Read the model definition and answer for the solid it produces. Units are mm, in the model's axes. Face numbers are marked on the shaded views. A direction names the side the tool comes from. Coordinates: 2 decimals unless noted, no trailing zeros. Order: outer loops, then holes, each group sorted by start corner. A loop starts at its lowest first (then second) coordinate and runs counter-clockwise, first axis right, second up. Notation, with made-up numbers: (73.25, -14) - (129.25, -14) arc R12 ccw to (129.25, -5) - close; hole circle Ø4 at (48.25, 29). An arc over 180 degrees is marked (long way). Write item = value, one per line.
from build123d import *

# Parameters (mm, degrees)
BOSS_EXTRUDE1_DEPTH = 38
SKETCH2_W           = 76
SKETCH2_H           = 2
BOSS_EXTRUDE2_DEPTH = 2
FILLET1_R           = 3
FILLET2_R           = 0.5
CUT_EXTRUDE1_REACH  = 57.31
SKETCH3_R           = 2
SKETCH4_W           = 74.032437302
SKETCH4_H           = 2
BOSS_EXTRUDE3_DEPTH = 0.35
FILLET3_R           = 0.25


with BuildPart() as part:
    # Sketch1 → Boss-Extrude1 (new body)
    with BuildSketch(Plane.XY):
        Polygon((35.755845082, 24), (37.016218651, 22.2), (-37.016218651, 22.2), (-35.755845082, 24), (-35.755845082, 24.1), (-38, 24.1), (-38, 26.1), (38, 26.1), (38, 24.1), (35.755845082, 24.1), align=None)
    extrude(amount=-BOSS_EXTRUDE1_DEPTH)

    # Sketch2 → Boss-Extrude2 (add)
    with BuildSketch(Plane(origin=(0, 0, -38), x_dir=(-1, 0, 0), z_dir=(0, 0, -1))):
        with Locations((0, 25.1)):
            Rectangle(SKETCH2_W, SKETCH2_H)
    extrude(amount=BOSS_EXTRUDE2_DEPTH)

    # Fillet1
    fillet1_edges = [part.edges().sort_by_distance(p)[0] for p in [
        (-38, 25.1, -40),
        (38, 25.1, -40),
    ]]
    fillet(fillet1_edges, radius=FILLET1_R)

    # Fillet2
    fillet2_edges = [part.edges().sort_by_distance(p)[0] for p in [
        (0, 26.1, 0),
        (-38, 26.1, -18.5),
        (0, 26.1, -40),
        (38, 26.1, -18.5),
        (37.121320344, 26.1, -39.121320344),
        (-37.121320344, 26.1, -39.121320344),
    ]]
    fillet(fillet2_edges, radius=FILLET2_R)

    # Sketch3 → Cut-Extrude1 (cut, up to next)
    with BuildSketch(Plane(origin=(0, 26.1, 0), x_dir=(1, 0, 0), z_dir=(0, 1, 0)), mode=Mode.PRIVATE) as cut_extrude1_sk1:
        with Locations(Location((-23, 20, 0), (0, 0, 270))):
            Circle(SKETCH3_R)
    cut_extrude1_tool1 = extrude(cut_extrude1_sk1.sketch, amount=-CUT_EXTRUDE1_REACH, mode=Mode.PRIVATE) & part.part
    # Sketch3 → Cut-Extrude1 (cut, up to next)
    with BuildSketch(Plane(origin=(0, 26.1, 0), x_dir=(1, 0, 0), z_dir=(0, 1, 0)), mode=Mode.PRIVATE) as cut_extrude1_sk2:
        with Locations(Location((23, 20, 0), (0, 0, 180))):
            Circle(SKETCH3_R)
    cut_extrude1_tool2 = extrude(cut_extrude1_sk2.sketch, amount=-CUT_EXTRUDE1_REACH, mode=Mode.PRIVATE) & part.part
    add(cut_extrude1_tool1.solids().sort_by_distance((-23, 26.1, -20))[0], mode=Mode.SUBTRACT)
    add(cut_extrude1_tool2.solids().sort_by_distance((23, 26.1, -20))[0], mode=Mode.SUBTRACT)

    # Sketch4 → Boss-Extrude3 (add)
    with BuildSketch(Plane.XZ.offset(-22.2)):
        with Locations((0, -2.5)):
            Rectangle(SKETCH4_W, SKETCH4_H)
    extrude(amount=BOSS_EXTRUDE3_DEPTH)

    # Fillet3
    fillet3_edges = [part.edges().sort_by_distance(p)[0] for p in [
        (0, 21.85, -1.5),
        (0, 21.85, -3.5),
    ]]
    fillet(fillet3_edges, radius=FILLET3_R)


solid = part.part
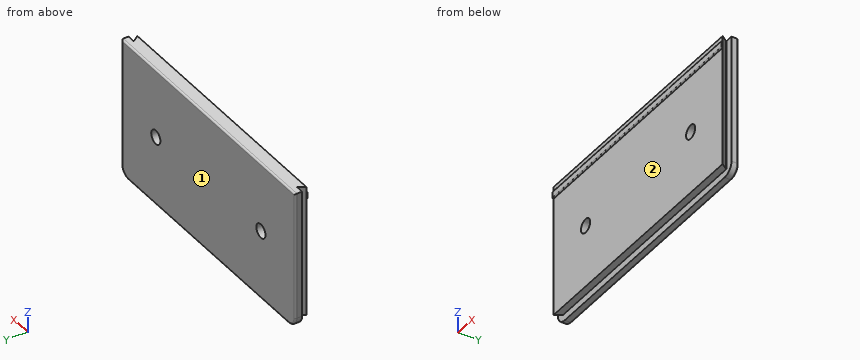
1) Straight lines are drawn through the part: line 1 along Y through (x, z) = (-3, -16); line 2 along Z through (x, y) = (-8.5, 23.5); line 3 along X through (y, z) = (23.35, -21.5). For each, find the intervals that lie inside material, in ascending order. Write a range as from..to.
Returned:
line_1 = 22.2..26.1
line_2 = -38..0
line_3 = -36.21..-24.32, -21.68..21.68, 24.32..36.21
2) The part is cut by section C-C (z = -34.5). Determine the outline of the cut face in (x, y).
Returned:
outline = (-38, 24.1) - (-35.76, 24.1) - (-35.76, 24) - (-37.02, 22.2) - (37.02, 22.2) - (35.76, 24) - (35.76, 24.1) - (38, 24.1) - (38, 25.6) arc R0.5 ccw to (37.5, 26.1) - (-37.5, 26.1) arc R0.5 ccw to (-38, 25.6) - close
3) The part is cut by section A-A (x = -23). Determine the outline of the cut face in (y, z), and give its area (3 significant figures).
Returned:
outline = (21.85, -3.25) arc R0.25 ccw to (22.1, -3.5) - (22.2, -3.5) - (22.2, -18) - (26.1, -18) - (26.1, -0.5) arc R0.5 ccw to (25.6, 0) - (22.2, 0) - (22.2, -1.5) - (22.1, -1.5) arc R0.25 ccw to (21.85, -1.75) - close; (22.2, -38) - (24.1, -38) - (24.1, -40) - (25.6, -40) arc R0.5 ccw to (26.1, -39.5) - (26.1, -22) - (22.2, -22) - close
area = 137 mm^2
4) For the marked faces 1 and 2, determine the directions among +Z, -Z, +X, -X, +Y, -Y from which every point of the face is accessible in a straight line to the end or side of a thin tool.
Returned:
face_1 = +Z, -Z, +X, -X, +Y
face_2 = -Z, +X, -X, -Y
5) The part is cut by section D-D (x = 7). Determine the outline of the cut face in (y, z), and give its area (3 significant figures).
Returned:
outline = (21.85, -3.25) arc R0.25 ccw to (22.1, -3.5) - (22.2, -3.5) - (22.2, -38) - (24.1, -38) - (24.1, -40) - (25.6, -40) arc R0.5 ccw to (26.1, -39.5) - (26.1, -0.5) arc R0.5 ccw to (25.6, 0) - (22.2, 0) - (22.2, -1.5) - (22.1, -1.5) arc R0.25 ccw to (21.85, -1.75) - close
area = 153 mm^2
6) Flat-ended cylindrical pins translate along their axes: pin 1 Ø10 at (x, z) = (6.5, -22.5) entering from -Y; pin 2 Ø1.5 at (y, z) = (23, -18) entering from -X; pin 3 Ø0.6 at (x, y) = (-14.5, 23.5) entering from -Z. Find the tip coordinate at first contact, or state that the pin passes through.
Returned:
pin_1 = 22.2
pin_2 = -36.98
pin_3 = -38
7) The part is cut by section B-B (z = -20). Determine the outline of the cut face in (x, y).
Returned:
outline = (-38, 24.1) - (-35.76, 24.1) - (-35.76, 24) - (-37.02, 22.2) - (-25, 22.2) - (-25, 26.1) - (-37.5, 26.1) arc R0.5 ccw to (-38, 25.6) - close; (-21, 22.2) - (21, 22.2) - (21, 26.1) - (-21, 26.1) - close; (25, 22.2) - (37.02, 22.2) - (35.76, 24) - (35.76, 24.1) - (38, 24.1) - (38, 25.6) arc R0.5 ccw to (37.5, 26.1) - (25, 26.1) - close
